from build123d import *

# Parameters (mm, degrees)
SKETCH1_W             = 10
SKETCH1_H             = 23
SKETCH1_R             = 1.25
SKETCH1_R_2           = 1.5
BOSS_EXTRUDE1_DEPTH   = 10
SKETCH1_H_2           = 7
SKETCH1_R_3           = 1.875
BOSS_EXTRUDE1_2_DEPTH = 10
SKETCH1_H_3           = 5.5
BOSS_EXTRUDE1_3_DEPTH = 10
FILLET1_R             = 4
SKETCH2_R             = 1.536328734
BOSS_EXTRUDE3_DEPTH   = 3.5
SKETCH3_W             = 10
SKETCH3_H             = 3.920500842
BOSS_EXTRUDE4_DEPTH   = 7.5
SKETCH4_W             = 10
SKETCH4_H             = 3.773973311
BOSS_EXTRUDE5_DEPTH   = 7.5
SKETCH5_R             = 1
CUT_EXTRUDE1_DEPTH    = 7


with BuildPart() as part:
    # Sketch1 → Boss-Extrude1 (new body)
    with BuildSketch(Plane.XY):
        with Locations((0, 10)):
            Rectangle(SKETCH1_W, SKETCH1_H)
        with Locations((-2.5, 12.5)):
            Circle(SKETCH1_R, mode=Mode.SUBTRACT)
        with Locations((0, 18.4)):
            Circle(SKETCH1_R_2, mode=Mode.SUBTRACT)
        with Locations((2.5, 12.5)):
            Circle(SKETCH1_R, mode=Mode.SUBTRACT)
    extrude(amount=BOSS_EXTRUDE1_DEPTH)

    # Fillet1
    fillet1_edges = [part.edges().sort_by_distance(p)[0] for p in [
        (-5, 21.5, 5),
        (5, 21.5, 5),
    ]]
    fillet(fillet1_edges, radius=FILLET1_R)

    # Sketch2 → Boss-Extrude3 (add)
    with BuildSketch(Plane(origin=(0, 0, 0), x_dir=(-1, 0, 0), z_dir=(0, 0, -1))):
        with Locations((0, 18.4)):
            Circle(SKETCH2_R)
    extrude(amount=-BOSS_EXTRUDE3_DEPTH)



with BuildPart() as body_2:
    # Sketch1 → Boss-Extrude1 2 (new body)
    with BuildSketch(Plane.XY):
        with Locations((0, -8.75)):
            Rectangle(SKETCH1_W, SKETCH1_H_2)
        with Locations((0, -8.75)):
            Circle(SKETCH1_R_3, mode=Mode.SUBTRACT)
    extrude(amount=BOSS_EXTRUDE1_2_DEPTH)


with BuildPart() as body_3:
    # Sketch1 → Boss-Extrude1 3 (new body)
    with BuildSketch(Plane.XY):
        with Locations((0, -18.75)):
            Rectangle(SKETCH1_W, SKETCH1_H_3)
    extrude(amount=BOSS_EXTRUDE1_3_DEPTH)


with BuildPart() as part_1:
    add(part.part)

    add(body_2.part)  # Boss-Extrude4 merges body 2
    # Sketch3 → Boss-Extrude4 (add)
    with BuildSketch(Plane(origin=(0, 0, 0), x_dir=(-1, 0, 0), z_dir=(0, 0, -1))):
        with Locations((0, -3.289749579)):
            Rectangle(SKETCH3_W, SKETCH3_H)
    extrude(amount=-BOSS_EXTRUDE4_DEPTH)


    add(body_3.part)  # Boss-Extrude5 merges body 3
    # Sketch4 → Boss-Extrude5 (add)
    with BuildSketch(Plane(origin=(0, 0, 0), x_dir=(-1, 0, 0), z_dir=(0, 0, -1))):
        with Locations((0, -14.113013345)):
            Rectangle(SKETCH4_W, SKETCH4_H)
    extrude(amount=-BOSS_EXTRUDE5_DEPTH)

    # Sketch5 → Cut-Extrude1 (cut)
    with BuildSketch(Plane.XZ.offset(21.5)):
        with Locations((0, 5)):
            Circle(SKETCH5_R)
    extrude(amount=-CUT_EXTRUDE1_DEPTH, mode=Mode.SUBTRACT)


solid = part_1.part
Could you check a few things on this model? Use its own coordinates, in mm. A direction names the side the tool comes from. Give positions to 0.01 mm unless a question says otherwise; leave off trailing zeros. Order: outer loops, then holes, each group sorted by start corner. A loop starts at its lowest first (then second) coordinate and runs counter-clockwise, first axis right, second up. Notation, with made-up numbers: (46, 3.25) -> (53, 3.25) arc R31 cw to (53, 31.25) -> close; hole circle Ø4 at (48.25, -33.5). An arc over 180 degrees is marked (long way). Answer in a Markdown table with one row per item. Add a question column.
Item 1: Please list where these lines run through material, in increasing order: probe 1 along Y at (x, z) = (0, 6.5) (3 decimals); probe 2 along X at (y, z) = (13, 3.75); probe 3 along Y at (x, z) = (-0.5, 7.75).
Item 2: For faces 4 (the flat face through (0, -14.5, 5)), 5 (the flat face through (0, -1.5, 9)), 6 (the flat face through (0, 21.5, 5)), 7 (the flat face through (0, -19, 10)), 8 (the cylindrical face through (-0.195, 19.887, 6.704)), which set-ups out of +Z, -Z, +X, -X, +Y, -Y let a thin tool reach every point of the face, with its end or its side?
Item 3: We'd pull the mould along X, two halves only. Please class faces 1 (the flat face through (0, -16, 9)), 2 (the cylindrical face through (-3.859, 20.297, 5.07)), 3 (the cylindrical face through (3.172, 13.554, 4.93)): pulls with the +X half, pulls with the -X half, needs draft (parallel to the pull), parting line crosses it, or undercut.
Item 4: Imagine slicing it at C-C (y = 12.5). List the corners of the cut face in (x, z) for me, and give its area (3 significant figures).
Item 5: I'm going to push a flat-ended pin straight in: P1, Ø1.1, axis at x = 1.5, y = -13.5, coming from the +Z side. Where does the tip first touch, or does it pass through?
Item 6: Imagine slicing it at A-A (z = 8). List the corners of the cut face in (x, y) for me (3 decimals).
Item 7: Imagine slicing it at D-D (z = 1.75). List the corners of the cut face in (x, y) for me (3 decimals).
Item 8: Imagine slicing it at B-B (x = 0). List the corners of the cut face in (y, z) for me (3 decimals), and give its area (3 significant figures).
Result:
| question | item | result |
|---|---|---|
| 1 | probe 1 | -21.5 to -10.625, -6.875 to 16.9, 19.9 to 21.5 |
| 1 | probe 2 | -5 to -3.65, -1.35 to 1.35, 3.65 to 5 |
| 1 | probe 3 | -21.5 to -16, -12.25 to -10.56, -6.94 to -5.25, -1.5 to 16.99, 19.81 to 21.5 |
| 2 | face 4 | -Y |
| 2 | face 5 | +Z, +X, -X |
| 2 | face 6 | +Z, -Z, +X, -X, +Y |
| 2 | face 7 | +Z, +X, -X, +Y, -Y |
| 2 | face 8 | +Z |
| 3 | face 1 | needs draft |
| 3 | face 2 | pulls with the -X half |
| 3 | face 3 | undercut |
| 4 | outline | (-5, 0) -> (-3.75, 0) -> (-3.75, 10) -> (-5, 10) -> close; (-1.25, 0) -> (1.25, 0) -> (1.25, 10) -> (-1.25, 10) -> close; (3.75, 0) -> (5, 0) -> (5, 10) -> (3.75, 10) -> close |
| 4 | area | 50.0 mm2 |
| 5 | P1 | z = 7.5 |
| 6 | outline | (-5, -21.5) -> (5, -21.5) -> (5, -16) -> (-5, -16) -> close; (-5, -12.25) -> (5, -12.25) -> (5, -5.25) -> (-5, -5.25) -> close; (-5, -1.5) -> (5, -1.5) -> (5, 17.5) arc R4 ccw to (1, 21.5) -> (-1, 21.5) arc R4 ccw to (-5, 17.5) -> close; hole circle Ø2.5 at (-2.5, 12.5); hole circle Ø3.75 at (0, -8.75); hole circle Ø3 at (0, 18.4); hole circle Ø2.5 at (2.5, 12.5) |
| 7 | outline | (-5, -21.5) -> (5, -21.5) -> (5, 17.5) arc R4 ccw to (1, 21.5) -> (-1, 21.5) arc R4 ccw to (-5, 17.5) -> close; hole circle Ø2.5 at (-2.5, 12.5); hole circle Ø3.75 at (0, -8.75); hole circle Ø2.5 at (2.5, 12.5) |
| 8 | outline | (-21.5, 0) -> (-10.625, 0) -> (-10.625, 10) -> (-12.25, 10) -> (-12.25, 7.5) -> (-16, 7.5) -> (-16, 10) -> (-21.5, 10) -> (-21.5, 6) -> (-14.5, 6) -> (-14.5, 4) -> (-21.5, 4) -> close; (-6.875, 0) -> (21.5, 0) -> (21.5, 10) -> (19.9, 10) -> (19.9, 3.5) -> (16.9, 3.5) -> (16.9, 10) -> (-1.5, 10) -> (-1.5, 7.5) -> (-5.25, 7.5) -> (-5.25, 10) -> (-6.875, 10) -> close |
| 8 | area | 340 mm2 |
